```python
from build123d import *

# Parameters (mm, degrees)
F1_DEPTH      = 15.24
F3_T          = -2.54
F5_ANGLE_BACK = 22.5
F5_ANGLE      = 45
F9_DEPTH      = 5.08
F10_W         = 17.78
F10_H         = 12.7
F11_DEPTH     = 15.241


with BuildPart() as f1:
    # F0 (on Top) → F1 (new body)
    with BuildSketch(Plane.XY):
        Polygon((-50.8, 101.6), (-12.7, 0), (12.7, 0), (50.8, 101.6), align=None)
    extrude(amount=F1_DEPTH)

    # F3
    f3_openings = [f1.faces().sort_by_distance(p)[0] for p in [
        (0, 60.96, 0),
    ]]
    offset(amount=F3_T, openings=f3_openings)

    # F4 (on plane+point) → F5 (revolve)
    with BuildSketch(Plane.YZ, mode=Mode.PRIVATE) as f5_sk:
        Polygon((21.3342867792, 101.6), (0, 0), (17.5560421489, 0), (34.7880832851, 82.0639282465), align=None)
    revolve(f5_sk.sketch.rotate(Axis((0, 0, 50.8), (0, 0, 1)), -F5_ANGLE_BACK), axis=Axis((0, 0, 50.8), (0, 0, 1)), revolution_arc=F5_ANGLE)

    # F8 (on plane+point) + F7 (on plane+point) → F9 (join)
    with BuildSketch(Plane.XY.offset(15.24)):
        Polygon((49.2891350908, 96.7381212808), (50.525897119, 101.6652725557), (30.205897119, 101.6652725557), align=None)
    with BuildSketch(Plane.XY.offset(15.24)):
        Polygon((-29.7071077564, 101.5182593561), (-50.0271077564, 101.5182593561), (-49.2234366628, 96.5022337608), align=None)
    extrude(amount=F9_DEPTH)

    # F10 (on plane+point) → F11 (cut, through all)
    with BuildSketch(Plane.XY.offset(15.24)):
        Polygon((17.78, 101.726842235), (0, 101.726842235), (0, 89.026842235), (0, 88.7915473778), (17.78, 88.7915473778), align=None)
        with Locations((-8.89, 95.376842235)):
            Rectangle(F10_W, F10_H)
    extrude(amount=-F11_DEPTH, mode=Mode.SUBTRACT)


solid = f1.part
```
For this review, take the finished solid that the model builds, in its own axes (mm). A direction names the side the tool comes from. Coordinates: 2 decimals unless noted, no trailing zeros. Loops run counter-clockwise (first coordinate to the right, second up) from the corner with the lowest first, then second, coordinate; pieces in that order, holes last.
1. Mouldability with a two-part tool opening along Y and no side actions: class faces 1 (the flat face through (-4.35, 10.5, 6.44)), 2 (the flat face through (-39.602, 98.975, 17.744)), 3 (the flat face through (28.784, 50.124, 6.261)), 4 (the flat face through (42, 100, 20.32)) as +Y half, -Y half, draft (parallel to the pull), parting line (faces both ways), or undercut.
2. For line 1 (Z direction, x = -19, y = 33.5); line 2 (Z direction, x = 30.5, y = 53.5); line 3 (X direction, y = 28, z = 83), list the stretches that pass through material, from the lowest coordinate up.
3. Add section D-D, the plane x = -35.5. Give the boundary of the cut face in (y, z).
4. Add section B-B, the plane x = 24.5. Give the boundary of the cut face in (y, z).
5. Add section A-A, the plane z = 7.5. Give the boundary of the cut face in (x, y).
6. For faces 5 (the flat face through (-7.184, 17.344, 59.025)), 6 (the flat face through (33, 99.06, 6)), 7 (the flat face through (-17.78, 99.4, 11.1)), 8 (the flat face through (7.184, 17.344, 59.025)), list the 3-axis set-ups (+Z, -Z, +X, -X, +Y, -Y) from which the entire face can be reached by the end or side of a thin tool; tool diameter is ignored.
7. Add section C-C, the plane y = 66. Give the boundary of the cut face in (x, z).
8. Insertion check: P1, Ø11, axis at x = 4, z = 6, coming from the +Y side; P2, Ø1.5, axis at x = 3.5, z = 14.5, coming from the +Y side; P3, Ø4, axis at x = -40, z = 18, coming from the +Y side; P4, Ø1, axis at x = 49.5, y = 98.5, coming from the -Z side. Each pin has a flat end and moves straight along its axis. Give the tip position at first contact, or say it passes through.
Result:
1. face 1: undercut
1. face 2: -Y half
1. face 3: undercut
1. face 4: draft
2. line 1: z = 12.7 to 15.24
2. line 2: z = 0 to 15.24
2. line 3: x = -11.6 to 11.6
3. outline: (60.8, 0) - (68.03, 0) - (68.03, 12.7) - (99.06, 12.7) - (99.06, 0) - (101.6, 0) - (101.6, 15.24) - (101.52, 15.24) - (101.52, 20.32) - (100.03, 20.32) - (100.03, 15.24) - (60.8, 15.24) - close
4. outline: (31.47, 0) - (38.7, 0) - (38.7, 12.7) - (99.06, 12.7) - (99.06, 0) - (101.6, 0) - (101.6, 15.24) - (31.47, 15.24) - close
5. outline: (-50.8, 101.6) - (-12.7, 0) - (12.7, 0) - (50.8, 101.6) - (17.78, 101.6) - (17.78, 99.06) - (47.13, 99.06) - (10.94, 2.54) - (1.05, 2.54) - (7.32, 17.67) arc R19.13 ccw to (-7.32, 17.67) - (-1.05, 2.54) - (-10.94, 2.54) - (-47.13, 99.06) - (-17.78, 99.06) - (-17.78, 101.6) - close
6. face 5: +Z, -X, -Y
6. face 6: -Z
6. face 7: +Z, -Z, +Y
6. face 8: +Z, +X, -Y
7. outline: (-37.45, 0) - (-34.74, 0) - (-34.74, 12.7) - (34.74, 12.7) - (34.74, 0) - (37.45, 0) - (37.45, 15.24) - (-37.45, 15.24) - close
8. P1: stops at y = 19.79
8. P2: stops at y = 88.79
8. P3: stops at y = 101.52
8. P4: stops at z = 0
